Could you check a few things on this model? Use its own coordinates, in mm. Face numbers are marked on the shaded views. A direction names the side the tool comes from. Give positions to 0.01 mm unless a question says otherwise; leave off trailing zeros. Order: outer loops, then holes, each group sorted by start corner. A loop starts at its lowest first (then second) coordinate and runs counter-clockwise, first axis right, second up. Notation, with made-up numbers: M 61,6.5 L 82,6.5 A11 cw 82,24.5 Z; hole C 0.25,-19.5 d10. An arc over 180 degrees is marked long. Use a Markdown table: item, result. Add a question column.
Item 1: Suppose I cut it at C-C on x = -12. Write out the boundary of the cut face in (y, z), plus the area to 3 significant figures.
Item 2: Suppose I cut it at D-D on y = 11.5. Write out the boundary of the cut face in (x, z), plus the area to 3 significant figures.
Item 3: If we mould it in two halves opening along Z, with no side actions, what happens to the marked faces 5, 6, 7 and 8? For each: released by +Z, released by -Z, zero draft, split by the parting line, or undercut.
Item 4: I'm going to push flat-ended pins straight in: pin 1 Ø3.5 at (x, y) = (-0.5, 13) entering from -Z; pin 2 Ø1.5 at (y, z) = (7, -21) entering from +X; pin 3 Ø4 at (x, y) = (4.5, 8) entering from -Z. Where does each tip first touch, or does it pass through?
Item 5: If I drill on L1, parallel to Y at x = 0, z = -1.2; L2, parallel to Y at x = -3.5, z = -5.5; L3, parallel to Z at x = -21, y = -7, over which ranges is the centre line in solid material (lowest first)? Write a range as from..to.
Item 6: Suppose I cut it at B-B on x = 0. Write out the boundary of the cut face in (y, z), plus the area to 3 significant figures.
Item 7: Suppose I cut it at A-A on y = -5.5. Write out the boundary of the cut face in (x, z).
Item 8: For the marked faces 1, 2, 3 and 4, which set-ups out of +Z, -Z, +X, -X, +Y, -Y let a thin tool reach every point of the face, with its end or its side?
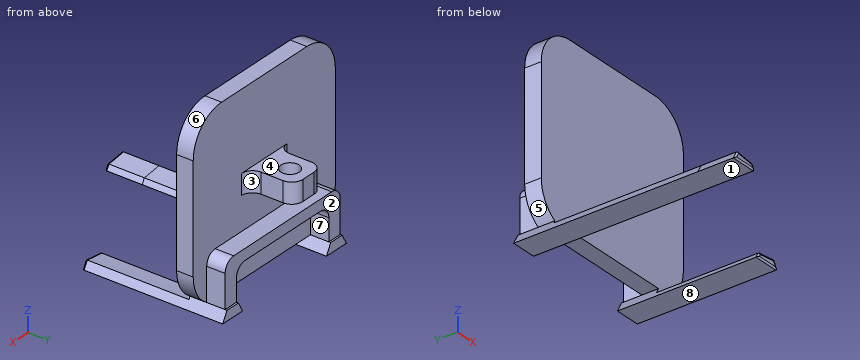
from build123d import *

# Parameters (mm, degrees)
EXTRUDE_1_DEPTH      = 4.5
EXTRUDE_2_DEPTH      = 40
EXTRUDE_2_DEPTH_BACK = 10
CUT_EXTRUDE_1_DEPTH  = 111
FILLET_1_R           = 10
SKETCH_4_W           = 16.25
SKETCH_4_H           = 3
EXTRUDE_3_DEPTH      = 5
FILLET_2_R           = 10
SKETCH_5_W           = 10
SKETCH_5_H           = 5.5
EXTRUDE_4_DEPTH      = 12
SKETCH_6_R           = 2.5
CUT_EXTRUDE_2_DEPTH  = 6
FILLET_3_R           = 3
FILLET_4_R           = 3
EXTRUDE_5_DEPTH      = 10
SKETCH_8_W           = 7
SKETCH_8_H           = 12
CUT_EXTRUDE_3_DEPTH  = 11.8
FILLET_5_R           = 0.4


with BuildPart() as part:
    # 草图1 → 凸台-拉伸1 (new body)
    with BuildSketch(Plane(origin=(0, 0, 0), x_dir=(1, 0, 0), z_dir=(0, 1, 0))):
        Polygon((-25, 23.7), (-25, -23.7), (25, -23.7), (25, 23.7), (20.25, 23.7), (21.75, 26.4), (14.75, 26.4), (16.25, 23.7), (-16.25, 23.7), (-14.75, 26.4), (-21.75, 26.4), (-20.25, 23.7), align=None)
    extrude(amount=EXTRUDE_1_DEPTH)

    # 草图2 → 凸台-拉伸2 (add, two sides: drawn at the far end of the back side and taken through both)
    with BuildSketch(Plane.XZ.offset(-EXTRUDE_2_DEPTH_BACK)):
        Polygon((-20.25, -23.7), (-16.25, -23.7), (-14.75, -26.4), (-21.75, -26.4), align=None)
        Polygon((16.25, -23.7), (20.25, -23.7), (21.75, -26.4), (14.75, -26.4), align=None)
    extrude(amount=EXTRUDE_2_DEPTH + EXTRUDE_2_DEPTH_BACK)

    # 草图3 → 切除-拉伸1 (cut)
    with BuildSketch(Plane.XZ):
        with BuildLine():
            Line((-25, -23.7), (25, -23.7))
            ThreePointArc((25, -23.7), (0, -25.88674251), (-25, -23.7))
        make_face()
    extrude(amount=CUT_EXTRUDE_1_DEPTH, mode=Mode.SUBTRACT)

    # 圆角1
    # the kernel refuses this fillet: 10 mm, written as the material it takes off along each edge
    with BuildSketch(Plane(origin=(25, -21.277555663, -23.7), x_dir=(0, 0, 1), z_dir=(0, 1, 0))) as fillet_1_piece_1:
        with BuildLine():
            CenterArc((8.511022265, -10), FILLET_1_R, 90, 58.331756746)
            Line((0, -4.75), (-0.170220445, -4.645))
            ThreePointArc((-0.170220445, -4.645), (-0.2, -2.375), (-0.2, 0))
            Line((-0.2, 0), (0, 0.2))
            Line((0, 0.2), (8.511022265, 0.2))
            Line((8.511022265, 0.2), (8.511022265, 0))
        make_face()
    extrude(amount=47.055111326, mode=Mode.SUBTRACT)
    with BuildSketch(Plane(origin=(-25, -21.277555663, -23.7), x_dir=(0, 0, 1), z_dir=(0, 1, 0))) as fillet_1_piece_2:
        with BuildLine():
            CenterArc((8.511022265, 10), FILLET_1_R, 211.668243254, 58.331756746)
            Line((0, 4.75), (-0.170220445, 4.645))
            ThreePointArc((-0.170220445, 4.645), (-0.2, 2.375), (-0.2, 0))
            Line((-0.2, 0), (0, -0.2))
            Line((0, -0.2), (8.511022265, -0.2))
            Line((8.511022265, -0.2), (8.511022265, 0))
        make_face()
    extrude(amount=47.055111326, mode=Mode.SUBTRACT)

    # 草图4 → 凸台-拉伸3 (add)
    with BuildSketch(Plane(origin=(0, 4.5, 0), x_dir=(1, 0, 0), z_dir=(0, 1, 0))):
        Polygon((-16.25, 23.7), (-20.25, 23.7), (-20.25, 11.7), (-16.25, 11.7), (-16.25, 14.7), align=None)
        with Locations((-8.125, 13.2)):
            Rectangle(SKETCH_4_W, SKETCH_4_H)
        with Locations((8.125, 13.2)):
            Rectangle(SKETCH_4_W, SKETCH_4_H)
        Polygon((16.25, 14.7), (16.25, 11.7), (20.25, 11.7), (20.25, 23.7), (16.25, 23.7), align=None)
    extrude(amount=EXTRUDE_3_DEPTH)

    # 圆角2
    fillet_2_edges = [part.edges().sort_by_distance(p)[0] for p in [
        (-25, 2.25, 23.7),
        (25, 2.25, 23.7),
    ]]
    fillet(fillet_2_edges, radius=FILLET_2_R)

    # 草图5 → 凸台-拉伸4 (add)
    with BuildSketch(Plane(origin=(0, 4.5, 0), x_dir=(1, 0, 0), z_dir=(0, 1, 0))):
        Rectangle(SKETCH_5_W, SKETCH_5_H)
    extrude(amount=EXTRUDE_4_DEPTH)

    # 草图6 → 切除-拉伸2 (cut)
    with BuildSketch(Plane.XY.offset(2.75)):
        with Locations((0, 11.5)):
            Circle(SKETCH_6_R)
    extrude(amount=-CUT_EXTRUDE_2_DEPTH, mode=Mode.SUBTRACT)

    # 圆角3
    fillet_3_edges = [part.edges().sort_by_distance(p)[0] for p in [
        (5, 4.5, 0),
        (-5, 4.5, 0),
        (5, 16.5, 0),
        (-5, 16.5, 0),
    ]]
    fillet(fillet_3_edges, radius=FILLET_3_R)

    # 圆角4
    fillet_4_edges = [part.edges().sort_by_distance(p)[0] for p in [
        (-16.25, 7, -14.7),
        (-20.25, 7, -11.7),
        (20.25, 7, -11.7),
        (16.25, 7, -14.7),
    ]]
    fillet(fillet_4_edges, radius=FILLET_4_R)

    # 草图7 → 凸台-拉伸5 (add)
    with BuildSketch(Plane.XZ.offset(40)):
        with BuildLine():
            Line((-14.75, -26.4), (-15.499934547, -25.050117816))
            ThreePointArc((-15.499934547, -25.050117816), (-18.072342022, -24.748180462), (-20.638902789, -24.400025019))
            Line((-20.638902789, -24.400025019), (-21.75, -26.4))
            Line((-21.75, -26.4), (-14.75, -26.4))
        make_face()
    extrude(amount=EXTRUDE_5_DEPTH)

    # 草图8 → 切除-拉伸3 (cut)
    with BuildSketch(Plane(origin=(0, 0, -26.4), x_dir=(-1, 0, 0), z_dir=(0, 0, -1))):
        with Locations((-18.25, -34)):
            Rectangle(SKETCH_8_W, SKETCH_8_H)
    extrude(amount=-CUT_EXTRUDE_3_DEPTH, mode=Mode.SUBTRACT)

    # 圆角5
    fillet_5_edges = [part.edges().sort_by_distance(p)[0] for p in [
        (-18.25, -50, -26.4),
        (-15.124967273, -50, -25.725058908),
        (-18.072342022, -50, -24.748180462),
        (-21.194451394, -50, -25.40001251),
        (18.072342022, -28, -24.748180462),
        (21.194451394, -28, -25.40001251),
        (15.124967273, -28, -25.725058908),
        (18.25, -28, -26.4),
    ]]
    fillet(fillet_5_edges, radius=FILLET_5_R)


solid = part.part
Findings below:
| question | item | result |
|---|---|---|
| 1 | outline | M 0,-23.7 L 4.5,-23.7 L 4.5,-14.7 L 9.5,-14.7 L 9.5,-11.7 L 4.5,-11.7 L 4.5,23.7 L 0,23.7 Z |
| 1 | area | 228 mm^2 |
| 2 | outline | M -5,-2.75 L -2.5,-2.75 L -2.5,2.75 L -5,2.75 Z; M 2.5,-2.75 L 5,-2.75 L 5,2.75 L 2.5,2.75 Z |
| 2 | area | 27.5 mm^2 |
| 3 | face 5 | undercut |
| 3 | face 6 | released by +Z |
| 3 | face 7 | undercut |
| 3 | face 8 | released by -Z |
| 4 | pin 1 | stops at z = -2.75 |
| 4 | pin 2 | stops at x = 20.25 |
| 4 | pin 3 | stops at z = -14.7 |
| 5 | L1 | y = 0..9, 14..16.5 |
| 5 | L2 | y = 0..4.5 |
| 5 | L3 | z = -26.4..-25.05 |
| 6 | outline | M 0,-23.7 L 4.5,-23.7 L 4.5,-14.7 L 9.5,-14.7 L 9.5,-11.7 L 4.5,-11.7 L 4.5,-2.75 L 9,-2.75 L 9,2.75 L 4.5,2.75 L 4.5,23.7 L 0,23.7 Z; M 14,-2.75 L 16.5,-2.75 L 16.5,2.75 L 14,2.75 Z |
| 6 | area | 267 mm^2 |
| 7 | outline | M -21.75,-26.4 L -14.75,-26.4 L -15.5,-25.05 A144 cw -20.64,-24.4 Z; M 14.75,-26.4 L 21.75,-26.4 L 20.64,-24.4 A144 cw 15.5,-25.05 Z |
| 8 | face 1 | -Z, +X, -X, +Y, -Y |
| 8 | face 2 | +X, -X, +Y |
| 8 | face 3 | +Z, +X, +Y |
| 8 | face 4 | +Z, +X, -X, +Y |
